```python
from build123d import *

# Parameters (mm, degrees)
MODEL_R                 = 1.5
P_IDAT_VYSUNUT_M1_DEPTH = 2.8


with BuildPart() as part:
    # Model → Přidat vysunutím1 (new body)
    with BuildSketch(Plane.XY):
        with BuildLine():
            Line((-14.2, 18.25), (14.2, 18.25))
            Line((14.2, 18.25), (15.610615846, 10.25))
            Line((15.610615846, 10.25), (16.010615846, 10.25))
            Line((16.010615846, 10.25), (14.071019058, 21.25))
            Line((14.071019058, 21.25), (12.101403552, 20.902703645))
            Line((12.101403552, 20.902703645), (11.893025739, 22.084472948))
            Line((11.893025739, 22.084472948), (14.706771698, 23.907401431))
            Line((14.706771698, 23.907401431), (15.892964362, 24.088914415))
            Line((15.892964362, 24.088914415), (18.010615846, 10.25))
            Line((18.010615846, 10.25), (18.9, 10.25))
            Line((18.9, 10.25), (18.9, 21.596640106))
            ThreePointArc((18.9, 21.596640106), (20.7, 22.05), (22.5, 21.596640106))
            Line((22.5, 21.596640106), (22.5, 10.25))
            Line((22.5, 10.25), (23.389384154, 10.25))
            Line((23.389384154, 10.25), (25.507035638, 24.088914415))
            Line((25.507035638, 24.088914415), (26.693228302, 23.907401431))
            Line((26.693228302, 23.907401431), (29.506974261, 22.084472948))
            Line((29.506974261, 22.084472948), (29.298596448, 20.902703645))
            Line((29.298596448, 20.902703645), (27.328980942, 21.25))
            Line((27.328980942, 21.25), (25.389384154, 10.25))
            Line((25.389384154, 10.25), (25.789384154, 10.25))
            Line((25.789384154, 10.25), (27.2, 18.25))
            Line((27.2, 18.25), (32.5, 18.25))
            Line((32.5, 18.25), (32.5, -18.25))
            Line((32.5, -18.25), (27.2, -18.25))
            Line((27.2, -18.25), (25.789384154, -10.25))
            Line((25.789384154, -10.25), (25.389384154, -10.25))
            Line((25.389384154, -10.25), (27.328980942, -21.25))
            Line((27.328980942, -21.25), (29.298596448, -20.902703645))
            Line((29.298596448, -20.902703645), (29.506974261, -22.084472948))
            Line((29.506974261, -22.084472948), (26.693228302, -23.907401431))
            Line((26.693228302, -23.907401431), (25.507035638, -24.088914415))
            Line((25.507035638, -24.088914415), (23.389384154, -10.25))
            Line((23.389384154, -10.25), (22.5, -10.25))
            Line((22.5, -10.25), (22.5, -21.596640106))
            ThreePointArc((22.5, -21.596640106), (20.7, -22.05), (18.9, -21.596640106))
            Line((18.9, -21.596640106), (18.9, -10.25))
            Line((18.9, -10.25), (18.010615846, -10.25))
            Line((18.010615846, -10.25), (15.892964362, -24.088914415))
            Line((15.892964362, -24.088914415), (14.706771698, -23.907401431))
            Line((14.706771698, -23.907401431), (11.893025739, -22.084472948))
            Line((11.893025739, -22.084472948), (12.101403552, -20.902703645))
            Line((12.101403552, -20.902703645), (14.071019058, -21.25))
            Line((14.071019058, -21.25), (16.010615846, -10.25))
            Line((16.010615846, -10.25), (15.610615846, -10.25))
            Line((15.610615846, -10.25), (14.2, -18.25))
            Line((14.2, -18.25), (3.5, -18.25))
            Line((3.5, -18.25), (3.5, -12.45))
            Line((3.5, -12.45), (-3.5, -12.45))
            Line((-3.5, -12.45), (-3.5, -18.25))
            Line((-3.5, -18.25), (-14.2, -18.25))
            Line((-14.2, -18.25), (-15.610615846, -10.25))
            Line((-15.610615846, -10.25), (-16.010615846, -10.25))
            Line((-16.010615846, -10.25), (-14.071019058, -21.25))
            Line((-14.071019058, -21.25), (-12.101403552, -20.902703645))
            Line((-12.101403552, -20.902703645), (-11.893025739, -22.084472948))
            Line((-11.893025739, -22.084472948), (-14.706771698, -23.907401431))
            Line((-14.706771698, -23.907401431), (-15.892964362, -24.088914415))
            Line((-15.892964362, -24.088914415), (-18.010615846, -10.25))
            Line((-18.010615846, -10.25), (-18.9, -10.25))
            Line((-18.9, -10.25), (-18.9, -21.596640106))
            ThreePointArc((-18.9, -21.596640106), (-20.7, -22.05), (-22.5, -21.596640106))
            Line((-22.5, -21.596640106), (-22.5, -10.25))
            Line((-22.5, -10.25), (-23.389384154, -10.25))
            Line((-23.389384154, -10.25), (-25.507035638, -24.088914415))
            Line((-25.507035638, -24.088914415), (-26.693228302, -23.907401431))
            Line((-26.693228302, -23.907401431), (-29.506974261, -22.084472948))
            Line((-29.506974261, -22.084472948), (-29.298596448, -20.902703645))
            Line((-29.298596448, -20.902703645), (-27.328980942, -21.25))
            Line((-27.328980942, -21.25), (-25.389384154, -10.25))
            Line((-25.389384154, -10.25), (-25.789384154, -10.25))
            Line((-25.789384154, -10.25), (-27.2, -18.25))
            Line((-27.2, -18.25), (-32.5, -18.25))
            Line((-32.5, -18.25), (-32.5, 18.25))
            Line((-32.5, 18.25), (-27.2, 18.25))
            Line((-27.2, 18.25), (-25.789384154, 10.25))
            Line((-25.789384154, 10.25), (-25.389384154, 10.25))
            Line((-25.389384154, 10.25), (-27.328980942, 21.25))
            Line((-27.328980942, 21.25), (-29.298596448, 20.902703645))
            Line((-29.298596448, 20.902703645), (-29.506974261, 22.084472948))
            Line((-29.506974261, 22.084472948), (-26.693228302, 23.907401431))
            Line((-26.693228302, 23.907401431), (-25.507035638, 24.088914415))
            Line((-25.507035638, 24.088914415), (-23.389384154, 10.25))
            Line((-23.389384154, 10.25), (-22.5, 10.25))
            Line((-22.5, 10.25), (-22.5, 21.596640106))
            ThreePointArc((-22.5, 21.596640106), (-20.7, 22.05), (-18.9, 21.596640106))
            Line((-18.9, 21.596640106), (-18.9, 10.25))
            Line((-18.9, 10.25), (-18.010615846, 10.25))
            Line((-18.010615846, 10.25), (-15.892964362, 24.088914415))
            Line((-15.892964362, 24.088914415), (-14.706771698, 23.907401431))
            Line((-14.706771698, 23.907401431), (-11.893025739, 22.084472948))
            Line((-11.893025739, 22.084472948), (-12.101403552, 20.902703645))
            Line((-12.101403552, 20.902703645), (-14.071019058, 21.25))
            Line((-14.071019058, 21.25), (-16.010615846, 10.25))
            Line((-16.010615846, 10.25), (-15.610615846, 10.25))
            Line((-15.610615846, 10.25), (-14.2, 18.25))
        make_face()
        with Locations((-8.75, 13.25)):
            Circle(MODEL_R, mode=Mode.SUBTRACT)
        with Locations(Location((8.75, 13.25, 0), (0, 0, 180))):
            Circle(MODEL_R, mode=Mode.SUBTRACT)
        with BuildLine():
            Line((2.875009535, -8.806924836), (5.5, 0))
            Line((5.5, 0), (3, 0))
            ThreePointArc((3, 0), (0, 3), (-3, 0))
            Line((-3, 0), (-5.5, 0))
            Line((-5.5, 0), (-2.875009535, -8.806924836))
            ThreePointArc((-2.875009535, -8.806924836), (0, -10.95), (2.875009535, -8.806924836))
        make_face(mode=Mode.SUBTRACT)
    extrude(amount=P_IDAT_VYSUNUT_M1_DEPTH)


solid = part.part
```
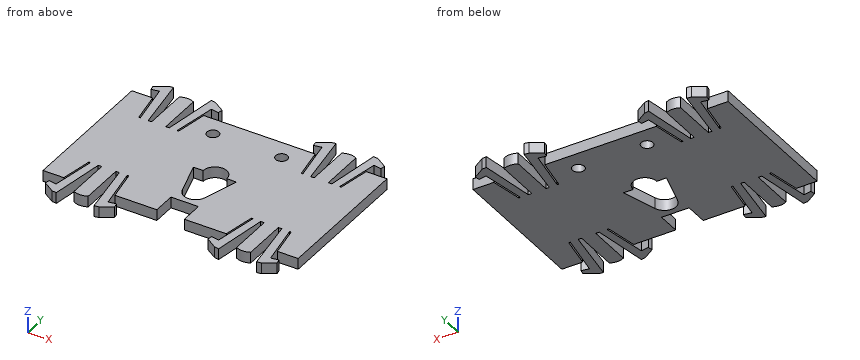
Geometry check sheet. Reference: the model listing, model coordinates, mm. Give positions to 0.01 mm unless a question says otherwise; leave off trailing zeros. Order: outer loops, then holes, each group sorted by start corner. A loop starts at its lowest first (then second) coordinate and runs counter-clockwise, first axis right, second up.
1. Gauge pin test, flat end, axial feed: pin 1 Ø0.7 at (x, z) = (23, 1.5) entering from -Y. Record the tip position at first contact, or that the pin passes through.
2. Section check C-C, the plane z = 1.65. Give the number of separate pieces and of enclosed holes in the cut face, and give its area (3 significant figures).
3. Thickness scan on L1, parallel to Y at x = 8.75, z = 2.1; L2, parallel to Y at x = 0, z = 0.9; L3, parallel to X at y = -4, z = 1.65. Record the ranges inside material, lowest first.
4. Section check D-D, the plane y = -19. Enter the section's corners in (x, z), and give its area (3 significant figures).
5. Section check B-B, the plane y = -1.5. Enter the section's corners in (x, z), and give its area (3 significant figures).
6. Section check A-A, the plane x = -8.75. Enter the section's corners in (y, z).
Values follow:
1. pin 1: stops at y = -10.25
2. separate pieces: 1
2. enclosed holes: 3
2. area: 2,280 mm2
3. L1: y = -18.25 to 11.75, 14.75 to 18.25
3. L2: y = -12.45 to -10.95, 3 to 18.25
3. L3: x = -32.5 to -4.31, 4.31 to 32.5
4. outline: (-26.93, 0) - (-24.73, 0) - (-24.73, 2.8) - (-26.93, 2.8) - close; (-22.5, 0) - (-18.9, 0) - (-18.9, 2.8) - (-22.5, 2.8) - close; (-16.67, 0) - (-14.47, 0) - (-14.47, 2.8) - (-16.67, 2.8) - close; (14.47, 0) - (16.67, 0) - (16.67, 2.8) - (14.47, 2.8) - close; (18.9, 0) - (22.5, 0) - (22.5, 2.8) - (18.9, 2.8) - close; (24.73, 0) - (26.93, 0) - (26.93, 2.8) - (24.73, 2.8) - close
4. area: 44.8 mm2
5. outline: (-32.5, 0) - (-5.05, 0) - (-5.05, 2.8) - (-32.5, 2.8) - close; (5.05, 0) - (32.5, 0) - (32.5, 2.8) - (5.05, 2.8) - close
5. area: 154 mm2
6. outline: (-18.25, 0) - (11.75, 0) - (11.75, 2.8) - (-18.25, 2.8) - close; (14.75, 0) - (18.25, 0) - (18.25, 2.8) - (14.75, 2.8) - close
